from build123d import *

# Parameters (mm, degrees)
F1_DEPTH = 3.55


with BuildPart() as f1:
    # F0 (on Front) → F1 (new body)
    with BuildSketch(Plane.XZ):
        with BuildLine():
            Line((12.9345, 11.7475), (-10.9855, 11.7475))
            ThreePointArc((-10.9855, 11.7475), (-12.781551, 11.003551), (-13.5255, 9.2075))
            Line((-13.5255, 9.2075), (-13.5255, 3.9844))
            Line((-13.5255, 3.9844), (-9.0581, 3.9844))
            Line((-9.0581, 3.9844), (-9.0581, 5.7769))
            ThreePointArc((-9.0581, 5.7769), (-7.6581, 7.1769), (-6.2581, 5.7769))
            Line((-6.2581, 5.7769), (-6.2581, 3.9844))
            Line((-6.2581, 3.9844), (-4.6893, 3.9844))
            Line((-4.6893, 3.9844), (-4.6893, 5.7769))
            ThreePointArc((-4.6893, 5.7769), (-3.2893, 7.1769), (-1.8893, 5.7769))
            Line((-1.8893, 5.7769), (-1.8893, 3.9844))
            Line((-1.8893, 3.9844), (-0.3205, 3.9844))
            Line((-0.3205, 3.9844), (-0.3205, 5.7769))
            ThreePointArc((-0.3205, 5.7769), (1.0795, 7.1769), (2.4795, 5.7769))
            Line((2.4795, 5.7769), (2.4795, 3.9844))
            Line((2.4795, 3.9844), (4.0483, 3.9844))
            Line((4.0483, 3.9844), (4.0483, 5.7769))
            ThreePointArc((4.0483, 5.7769), (5.4483, 7.1769), (6.8483, 5.7769))
            Line((6.8483, 5.7769), (6.8483, 3.9844))
            Line((6.8483, 3.9844), (15.4745, 3.9844))
            Line((15.4745, 3.9844), (15.4745, 9.2075))
            ThreePointArc((15.4745, 9.2075), (14.730551, 11.003551), (12.9345, 11.7475))
        make_face()
    extrude(amount=F1_DEPTH)


solid = f1.part
Here's how the part is built. I have some questions about the finished solid (model axes, mm). A direction names the side the tool comes from. Give positions to 0.01 mm unless a question says otherwise; leave off trailing zeros. Loops run counter-clockwise (first coordinate to the right, second up) from the corner with the lowest first, then second, coordinate; pieces in that order, holes last. Notation, with made-up numbers: (0, -7.5) -> (34, -7.5) arc R18 cw to (34, 21.5) -> close; hole circle Ø1 at (48, -15.5). An arc over 180 degrees is marked (long way). Answer as a JSON object with one key per item and string values. Group by question number.
Item 1: Imagine slicing it at A-A on z = 5.5. Write out the boundary of the cut face in (x, y).
Item 2: I need wall thicknesses on L1, parallel to X at y = -2, z = 5.75; L2, parallel to X at y = -2, z = 6.75; L3, parallel to Z at x = -3.5, y = -1. Which ranges of each line are inside material? Lowest first, please.
Item 3: On a 3-axis mill with a long thin cutter (end or side, diameter ignored), from which of +Z, -Z, +X, -X, +Y, -Y can I reach the whole of each face in a straight line? I mean faces 1 (the flat face through (1, -2, 11.748)), 2 (the flat face through (-9.058, -2, 5)). Say none if no direction works.
Item 4: Imagine slicing it at B-B on y = -0.45. Write out the boundary of the cut face in (x, z), then the cut area to 3 significant figures.
Item 5: Imagine slicing it at C-C on x = -4. Write out the boundary of the cut face in (y, z).
Item 6: Imagine slicing it at D-D on x = 0.75. Write out the boundary of the cut face in (y, z).
Answer list:
{
 "1": {"outline": "(-13.53, -3.55) -> (-9.06, -3.55) -> (-9.06, 0) -> (-13.53, 0) -> close; (-6.26, -3.55) -> (-4.69, -3.55) -> (-4.69, 0) -> (-6.26, 0) -> close; (-1.89, -3.55) -> (-0.32, -3.55) -> (-0.32, 0) -> (-1.89, 0) -> close; (2.48, -3.55) -> (4.05, -3.55) -> (4.05, 0) -> (2.48, 0) -> close; (6.85, -3.55) -> (15.47, -3.55) -> (15.47, 0) -> (6.85, 0) -> close"},
 "2": {"L1": "x = -13.53 to -9.06, -6.26 to -4.69, -1.89 to -0.32, 2.48 to 4.05, 6.85 to 15.47", "L2": "x = -13.53 to -8.66, -6.65 to -4.3, -2.28 to 0.07, 2.09 to 4.44, 6.45 to 15.47", "L3": "z = 7.16 to 11.75"},
 "3": {"face 1": "+Z, +X, -X, +Y, -Y", "face 2": "-Z, +Y, -Y"},
 "4": {"outline": "(-13.53, 3.98) -> (-9.06, 3.98) -> (-9.06, 5.78) arc R1.4 cw to (-6.26, 5.78) -> (-6.26, 3.98) -> (-4.69, 3.98) -> (-4.69, 5.78) arc R1.4 cw to (-1.89, 5.78) -> (-1.89, 3.98) -> (-0.32, 3.98) -> (-0.32, 5.78) arc R1.4 cw to (2.48, 5.78) -> (2.48, 3.98) -> (4.05, 3.98) -> (4.05, 5.78) arc R1.4 cw to (6.85, 5.78) -> (6.85, 3.98) -> (15.47, 3.98) -> (15.47, 9.21) arc R2.54 ccw to (12.93, 11.75) -> (-10.99, 11.75) arc R2.54 ccw to (-13.53, 9.21) -> close", "area": "190 mm2"},
 "5": {"outline": "(-3.55, 6.98) -> (0, 6.98) -> (0, 11.75) -> (-3.55, 11.75) -> close"},
 "6": {"outline": "(-3.55, 7.14) -> (0, 7.14) -> (0, 11.75) -> (-3.55, 11.75) -> close"}
}
